Verification items for the finished model (mm, model axes). Face numbers are marked on the shaded views. A direction names the side the tool comes from. Coordinates: 2 decimals unless noted, no trailing zeros. Loops run counter-clockwise (first coordinate to the right, second up) from the corner with the lowest first, then second, coordinate; pieces in that order, holes last. Notation, with made-up numbers: (55.25, -24.5) -> (80.25, -24.5) arc R23 ccw to (80.25, 11.5) -> close; hole circle Ø6 at (-31, 42.5). An arc over 180 degrees is marked (long way). Answer as a JSON object with one key per item and string values. Group by question number.
Q1. Cross-section at C-C on x = 8.25. Record the boundary of the cut face in (y, z).
Q2. Scan lines: L1, parallel to X at y = 2.5, z = -2.5 (3 decimals); L2, parallel to X at y = 3.75, z = -2; L3, parallel to Z at x = 18, y = 3. Record each from-to range of solid material in increasing order.
Q3. Cross-section at B-B on y = 5.75. Record the boundary of the cut face in (x, z) (3 decimals), and give its area (3 significant figures).
Q4. Set-up check for the marked faces 1, 2, 3, 4 and 5: record each of +Z, -Z, +X, -X, +Y, -Y from which the full face is reachable in a straight line by a thin tool's end or side.
Q5. Cross-section at A-A on z = -2.5. Record the boundary of the cut face in (x, y) (3 decimals), and give its area (3 significant figures).
Q6. Gauge pin test, flat ends, axial feed: pin 1 Ø1.9 at (y, z) = (4, -5) entering from +X; pin 2 Ø3.5 at (y, z) = (3, 3) entering from -X; pin 3 Ø0.9 at (x, y) = (4.5, 3.5) entering from +Z. Record the tip position at first contact, or that the pin passes through.
Q7. Release check for a two-part mould opening along X. For the marked faces 6, 7 and 8 record: released by +X, released by -X, zero draft, split by the parting line, or undercut.
Q8. Cross-section at D-D on x = 14.6. Record the boundary of the cut face in (y, z) (3 decimals), and give its area (3 significant figures).
```python
from build123d import *

# Parameters (mm, degrees)
SKETCH_1_W             = 19.8
SKETCH_1_H             = 10.2
EXTRUDE_1_DEPTH        = 6.4
CUT_EXTRUDE_1_REACH    = 25.174
SKETCH_2_R             = 1.175
EXTRUDE_1_2_DEPTH      = 1.8
EXTRUDE_1_2_DEPTH_BACK = 1.8
EXTRUDE_2_DEPTH        = 1.6
EXTRUDE_2_DEPTH_BACK   = 1.6
SKETCH_4_W             = 0.5
SKETCH_4_H             = 3.9
SKETCH_5_W             = 3
SKETCH_5_H             = 0.4
EXTRUDE_2_2_DEPTH      = 6.4


with BuildPart() as part:
    # 草图1 → Extrude 1 (new body)
    with BuildSketch(Plane(origin=(0, 0, 0), x_dir=(1, 0, 0), z_dir=(0, 1, 0))):
        with Locations((9.9, 5.1)):
            Rectangle(SKETCH_1_W, SKETCH_1_H)
    extrude(amount=EXTRUDE_1_DEPTH)

    # 草图2 → 切除-拉伸1 (cut, up to next)
    with BuildSketch(Plane(origin=(0, 6.4, 0), x_dir=(1, 0, 0), z_dir=(0, 1, 0)), mode=Mode.PRIVATE) as cut_extrude_1_sk1:
        with Locations(Location((5.1, 2.5, 0), (0, 0, 270))):
            Circle(SKETCH_2_R)
    cut_extrude_1_tool1 = extrude(cut_extrude_1_sk1.sketch, amount=-CUT_EXTRUDE_1_REACH, mode=Mode.PRIVATE) & part.part
    # 草图2 → 切除-拉伸1 (cut, up to next)
    with BuildSketch(Plane(origin=(0, 6.4, 0), x_dir=(1, 0, 0), z_dir=(0, 1, 0)), mode=Mode.PRIVATE) as cut_extrude_1_sk2:
        with Locations(Location((14.6, 2.5, 0), (0, 0, 270))):
            Circle(SKETCH_2_R)
    cut_extrude_1_tool2 = extrude(cut_extrude_1_sk2.sketch, amount=-CUT_EXTRUDE_1_REACH, mode=Mode.PRIVATE) & part.part
    add(cut_extrude_1_tool1.solids().sort_by_distance((5.1, 6.4, -2.5))[0], mode=Mode.SUBTRACT)
    add(cut_extrude_1_tool2.solids().sort_by_distance((14.6, 6.4, -2.5))[0], mode=Mode.SUBTRACT)

    # 草图3 → Extrude 1 2 (add, two sides: drawn at the far end of the back side and taken through both)
    with BuildSketch(Plane(origin=(0, 3.2, 0), x_dir=(1, 0, 0), z_dir=(0, 1, 0)).offset(-EXTRUDE_1_2_DEPTH_BACK)):
        with BuildLine():
            Line((2.403782047, 10.2), (2.403782047, 10.9))
            ThreePointArc((2.403782047, 10.9), (2.652741283, 11.501040764), (3.253782047, 11.75))
            Line((3.253782047, 11.75), (18.828768482, 11.75))
            ThreePointArc((18.828768482, 11.75), (19.440119445, 11.925962013), (19.864384241, 12.4))
            ThreePointArc((19.864384241, 12.4), (21.156458454, 13.021039277), (22.05, 11.9))
            Line((22.05, 11.9), (22.35, 11.9))
            ThreePointArc((22.35, 11.9), (21.223360659, 13.313484306), (19.594223608, 12.530434783))
            ThreePointArc((19.594223608, 12.530434783), (19.280636585, 12.180058879), (18.828768482, 12.05))
            Line((18.828768482, 12.05), (3.253782047, 12.05))
            ThreePointArc((3.253782047, 12.05), (2.440609249, 11.713172798), (2.103782047, 10.9))
            Line((2.103782047, 10.9), (2.103782047, 10.2))
            Line((2.103782047, 10.2), (2.403782047, 10.2))
        make_face()
    extrude(amount=EXTRUDE_1_2_DEPTH + EXTRUDE_1_2_DEPTH_BACK)

    # 草图4 → Extrude 2 (add, two sides: drawn at the far end of the back side and taken through both)
    with BuildSketch(Plane(origin=(0, 3.2, 0), x_dir=(1, 0, 0), z_dir=(0, 1, 0)).offset(-EXTRUDE_2_DEPTH_BACK)):
        with Locations((1.6, -1.95)):
            Rectangle(SKETCH_4_W, SKETCH_4_H)
        with Locations((10.4, -1.95)):
            Rectangle(SKETCH_4_W, SKETCH_4_H)
        with Locations((17.95, -1.95)):
            Rectangle(SKETCH_4_W, SKETCH_4_H)
    extrude(amount=EXTRUDE_2_DEPTH + EXTRUDE_2_DEPTH_BACK)

    # 草图5 → Extrude 2 2 (add)
    with BuildSketch(Plane(origin=(0, 6.4, 0), x_dir=(1, 0, 0), z_dir=(0, 1, 0))):
        with Locations((5.1, -0.2)):
            Rectangle(SKETCH_5_W, SKETCH_5_H)
        with Locations((14.6, -0.2)):
            Rectangle(SKETCH_5_W, SKETCH_5_H)
    extrude(amount=-EXTRUDE_2_2_DEPTH)


solid = part.part
```
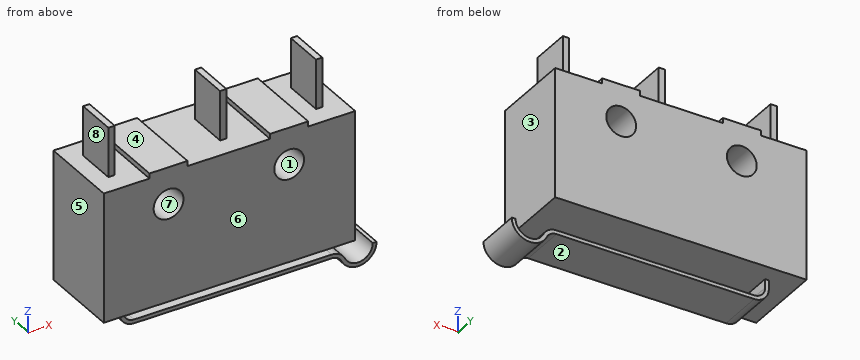
Computed values:
{
 "1": {"outline": "(0, -10.2) -> (6.4, -10.2) -> (6.4, 0) -> (0, 0) -> close; (1.4, -12.05) -> (5, -12.05) -> (5, -11.75) -> (1.4, -11.75) -> close"},
 "2": {"L1": "x = 0 to 3.925, 6.275 to 13.425, 15.775 to 19.8", "L2": "x = 0 to 4.04, 6.16 to 13.54, 15.66 to 19.8", "L3": "z = -12.05 to -11.75, -10.2 to 3.9"},
 "3": {"outline": "(0, -10.2) -> (19.8, -10.2) -> (19.8, 0) -> (16.1, 0) -> (16.1, 0.4) -> (13.1, 0.4) -> (13.1, 0) -> (6.6, 0) -> (6.6, 0.4) -> (3.6, 0.4) -> (3.6, 0) -> (0, 0) -> close; hole circle Ø2.35 at (5.1, -2.5); hole circle Ø2.35 at (14.6, -2.5)", "area": "196 mm²"},
 "4": {"face 1": "+Y, -Y", "face 2": "-Z, -X, +Y, -Y", "face 3": "+Z, +X, +Y, -Y", "face 4": "+Z, +Y, -Y", "face 5": "+Z, -Z, -X, +Y, -Y"},
 "5": {"outline": "(0, 0) -> (3.925, 0) -> (3.925, 6.4) -> (0, 6.4) -> close; (6.275, 0) -> (13.425, 0) -> (13.425, 6.4) -> (6.275, 6.4) -> close; (15.775, 0) -> (19.8, 0) -> (19.8, 6.4) -> (15.775, 6.4) -> close", "area": "96.6 mm²"},
 "6": {"pin 1": "stops at x = 19.8", "pin 2": "stops at x = 1.35", "pin 3": "stops at z = 0.4"},
 "7": {"face 6": "zero draft", "face 7": "undercut", "face 8": "released by -X"},
 "8": {"outline": "(0, -10.2) -> (6.4, -10.2) -> (6.4, -3.675) -> (0, -3.675) -> close; (0, -1.325) -> (6.4, -1.325) -> (6.4, 0.4) -> (0, 0.4) -> close; (1.4, -12.05) -> (5, -12.05) -> (5, -11.75) -> (1.4, -11.75) -> close", "area": "53.9 mm²"}
}
